Geometry: see drawing. Coordinates: mm, zero at the bounding-box minimum. A direction names the side the tool comes from. Coordinates: 2 decimals unless noted, no trailing zeros. Write each loop counter-clockwise with the first axis right and the second up, starting at its lowest first coordinate (ties: lowest second). Pieces come first, ordered by that corner, then holes. Notation, with made-up numbers: (54, -23) - (107, -23) arc R14 ccw to (107, 3) - close; hole circle Ø1 at (-18, 24.5). An arc over 180 degrees is marked (long way). One line per question, with ' | ' between items. Start each with the question number.
Q1. Draft query along Z for the marked faces 1, 2 and 3. Return one class per face: +Z half, -Z half, draft (parallel to the pull), parting line (faces both ways), or undercut.
Q2. Cut plane C-C, the plane y = 1.65. Return loops of the section in (x, z), plus the area to 3 significant figures.
Q3. Contact query for flat-ended pins moving along their axis: P1, Ø1.5, axis at y = 1, z = 6, coming from the -X side; P2, Ø0.6, axis at y = 3.5, z = 0.5, coming from the +X side; P3, Ø1.5, axis at x = 3, y = 3.5, coming from the +Z side; P4, Ø0.6, axis at y = 4, z = 7.5, coming from the -X side. Output: stop coordinate, or through.
Q4. Cut plane B-B, the plane z = 6.5. Return loops of the section in (x, y).
Q5. Line query: line 1 (Z direction, x = 5, y = 2.75); line 2 (Y direction, x = 3, z = 5.25); line 3 (X direction, y = 3.15, z = 0.75). Output: solid intervals per line, ascending.
Q6. Access query for the marked faces 4, 5 and 6. Directions: +Z, -Z, +X, -X, +Y, -Y. A direction counts if a zero-diameter tool reaches every point of the face in a straight line with its end or side. Return the directions, or none.
Q7. Cut plane A-A, the plane y = 3.15. Return loops of the section in (x, z).
Q8. Cut plane D-D, the plane x = 9. Return loops of the section in (y, z), plus the area to 4 significant figures.
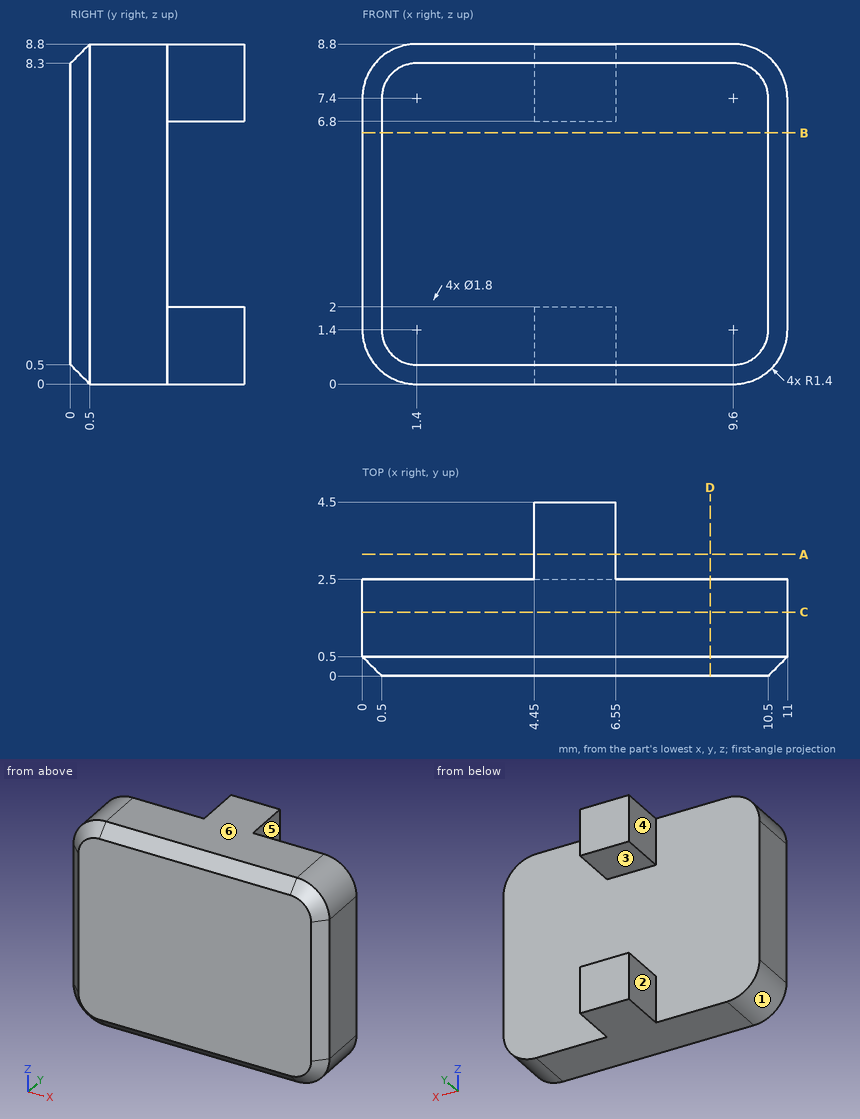
Reply:
1) face 1: -Z half | face 2: draft | face 3: undercut
2) outline: (0, 1.4) arc R1.4 ccw to (1.4, 0) - (9.6, 0) arc R1.4 ccw to (11, 1.4) - (11, 7.4) arc R1.4 ccw to (9.6, 8.8) - (1.4, 8.8) arc R1.4 ccw to (0, 7.4) - close | area: 95.1 mm^2
3) P1: stops at x = 0 | P2: stops at x = 6.55 | P3: passes through | P4: stops at x = 4.45
4) outline: (0, 0.5) - (0.5, 0) - (10.5, 0) - (11, 0.5) - (11, 2.5) - (0, 2.5) - close
5) line 1: z = 0 to 2, 6.8 to 8.8 | line 2: y = 0 to 2.5 | line 3: x = 4.45 to 6.55
6) face 4: +Z, -Z, -X, +Y | face 5: +Z, -Z, +X, +Y | face 6: +Z, +X, -X, +Y, -Y
7) outline: (4.45, 0) - (6.55, 0) - (6.55, 2) - (4.45, 2) - close; (4.45, 6.8) - (6.55, 6.8) - (6.55, 8.8) - (4.45, 8.8) - close
8) outline: (0, 0.5) - (0.5, 0) - (2.5, 0) - (2.5, 8.8) - (0.5, 8.8) - (0, 8.3) - close | area: 21.75 mm^2
